Read the model definition and answer for the solid it produces. Units are mm, in the model's axes. Coordinates: 2 decimals unless noted, no trailing zeros. Use a Markdown table: item, result.
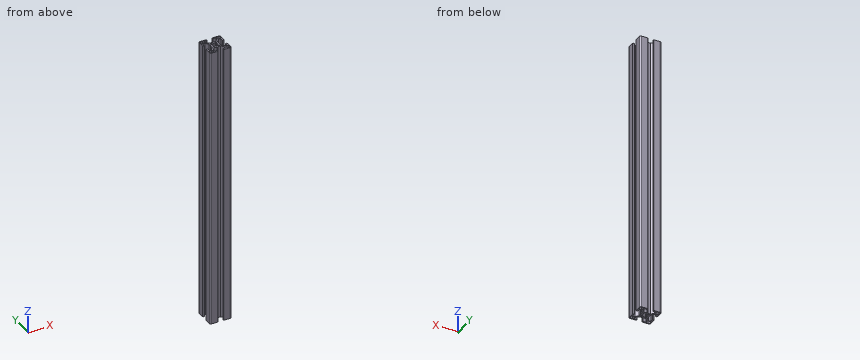
from build123d import *

# Parameters (mm, degrees)
BOSS_EXTRUDE1_DEPTH     = 200
CUT_EXTRUDE1_DEPTH      = 1
CUT_EXTRUDE1_DEPTH_BACK = 401


with BuildPart() as part:
    # Sketch4 → Boss-Extrude1 (new body, symmetric)
    with BuildSketch(Plane.XY):
        with BuildLine():
            Line((0, -5.45), (0.655464476, -6))
            Line((0.655464476, -6), (4.504469158, -6))
            Line((4.504469158, -6), (8.25, -9.745530842))
            Line((8.25, -9.745530842), (8.25, -12.885))
            Line((8.25, -12.885), (4, -12.885))
            Line((4, -12.885), (4, -14.45))
            Line((4, -14.45), (4.55, -14.45))
            Line((4.55, -14.45), (4.55, -15))
            Line((4.55, -15), (12.885, -15))
            ThreePointArc((12.885, -15), (14.380530842, -14.380530842), (15, -12.885))
            Line((15, -12.885), (15, -4.55))
            Line((15, -4.55), (14.45, -4.55))
            Line((14.45, -4.55), (14.45, -4))
            Line((14.45, -4), (12.885, -4))
            Line((12.885, -4), (12.885, -8.25))
            Line((12.885, -8.25), (9.745530842, -8.25))
            Line((9.745530842, -8.25), (6, -4.504469158))
            Line((6, -4.504469158), (6, -0.655464476))
            Line((6, -0.655464476), (5.45, 0))
            Line((5.45, 0), (3.5, 0))
            ThreePointArc((3.5, 0), (3.371433308, -0.939913534), (2.995178599, -1.81077474))
            Line((2.995178599, -1.81077474), (4.675743591, -3.491339732))
            Line((4.675743591, -3.491339732), (3.491339732, -4.675743591))
            Line((3.491339732, -4.675743591), (1.81077474, -2.995178599))
            ThreePointArc((1.81077474, -2.995178599), (0.939913534, -3.371433308), (0, -3.5))
            Line((0, -3.5), (0, -5.45))
        make_face()
        with BuildLine():
            Line((9.375, -10.365), (9.375, -12.885))
            ThreePointArc((9.375, -12.885), (9.664964287, -13.585035713), (10.365, -13.875))
            Line((10.365, -13.875), (12.885, -13.875))
            ThreePointArc((12.885, -13.875), (13.585035713, -13.585035713), (13.875, -12.885))
            Line((13.875, -12.885), (13.875, -10.365))
            ThreePointArc((13.875, -10.365), (13.585035713, -9.664964287), (12.885, -9.375))
            Line((12.885, -9.375), (10.365, -9.375))
            ThreePointArc((10.365, -9.375), (9.664964287, -9.664964287), (9.375, -10.365))
        make_face(mode=Mode.SUBTRACT)
    extrude(amount=BOSS_EXTRUDE1_DEPTH, both=True)

    # Mirror1: part across plane


with BuildPart() as part_1:
    add(part.part)
    add(part.part.mirror(Plane(origin=(0, 0, 0), x_dir=(0, 0, 1), z_dir=(1, 0, 0))))

    # Mirror2: part across plane


with BuildPart() as part_2:
    add(part_1.part)
    add(part_1.part.mirror(Plane.ZX))

    # Sketch5 → Cut-Extrude1 (cut, two sides)
    with BuildSketch(Plane.XY.offset(200)) as cut_extrude1_sk:
        Polygon((-5.675, 12.885), (-5.4, 13.16), (-5.125, 12.885), align=None)
    extrude(amount=CUT_EXTRUDE1_DEPTH, mode=Mode.SUBTRACT)
    extrude(cut_extrude1_sk.sketch, amount=-CUT_EXTRUDE1_DEPTH_BACK, mode=Mode.SUBTRACT)


solid = part_2.part
(1) A cutting plane is placed at A-A, the plane z = 18. Count the separate pieces of the cut face and the enclosed holes in it, and give its area (3 significant figures).
Report:
| item | result |
|---|---|
| separate pieces | 1 |
| enclosed holes | 5 |
| area | 295 mm² |
(2) Straight lines are drawn through the part: L1, parallel to Y at x = -13, z = 88; L2, parallel to X at y = -11.25, z = -43.5 (3 decimals); L3, parallel to X at y = 10, z = -8. For each, find the intervals that lie inside material, in ascending order.
Report:
| item | result |
|---|---|
| L1 | y = -15 to -13.87, -9.38 to -4, 4 to 9.38, 13.87 to 15 |
| L2 | x = -15 to -13.875, -9.375 to -8.25, 8.25 to 9.375, 13.875 to 15 |
| L3 | x = -15 to -13.81, -9.44 to -8.25, 8.25 to 9.44, 13.81 to 15 |
(3) Each of these flat-tipped pins is pushed along its axis until it touches: P1, Ø0.8, axis at x = 14, z = -43, coming from the +Y side; P2, Ø0.8, axis at y = 14, z = -56.5, coming from the -X side; P3, Ø2, axis at x = 8, y = 1, coming from the -Z side (1 decimal); P4, Ø0.8, axis at x = -13.5, z = 50.5, coming from the -Y side. Where does it stop, or does it pass through?
Report:
| item | result |
|---|---|
| P1 | stops at y = 14.88 |
| P2 | stops at x = -14.88 |
| P3 | passes through |
| P4 | stops at y = -14.99 |
